Design review of the part built by this model. Coordinates are the model's own, in mm. A direction names the side the tool comes from. Coordinates: 2 decimals unless noted, no trailing zeros. Write each loop counter-clockwise with the first axis right and the second up, starting at its lowest first coordinate (ties: lowest second). Pieces come first, ordered by that corner, then holes. Notation, with made-up numbers: (-18, 43) -> (-10, 43) arc R20 ccw to (-10, 49) -> close; hole circle Ø1 at (7, -6.5). An arc over 180 degrees is marked (long way). Answer in a Markdown table with one row per item. Add a question column.
Item 1: Take a section at A-A, the plane z = -6.5. Write out the cut boundary in (x, y), and give its area (3 significant figures).
Item 2: Draft analysis for pull direction X (two halves, no side actions). For faces 4 (the face through (18.374, 39, 14)), 5 (the face through (20.374, 21, 16)), 6 (the face through (0.4, 80, -8.3)), 7 (the face through (1, 39, -7.879)), state which applies: released by +X, released by -X, zero draft, split by the parting line, or undercut.
Item 3: For faces 1 (the face through (19.39, 24.35, 11.92)), 2 (the face through (-17.283, 39, 13)), 3 (the face through (-24.283, 39, 10)), list the 3-axis set-ups (+Z, -Z, +X, -X, +Y, -Y) from which the entire face can be reached by the end or side of a thin tool; tool diameter is ignored.
Item 4: Clearance check with flat-ended pins moving along their axes: P1, Ø10.5, axis at x = -4, y = 24.5, coming from the +Z side; P2, Ø7.5, axis at y = 18, z = 13.5, coming from the +X side; P3, Ø9, axis at y = 18.63, z = 10.12, coming from the +X side. State where each tip first meets the part, or that it passes through.
Item 5: Take a section at C-C, the plane x = -7. Write out the cut boundary in (y, z), and give its area (3 significant figures).
Item 6: To check wall thickness, follow line 1 (X direction, y = 51, z = 9); line 2 (Z direction, x = -2.5, y = 8). State the ranges of each line that lie inside material, in increasing order.
Item 7: Take a section at B-B, the plane y = 32.5. Write out the cut boundary in (x, z), and give its area (3 significant figures).
from build123d import *

# Parameters (mm, degrees)
F1_DEPTH = 80
F2_R     = 6
F3_DEPTH = 25
F2_R_2   = 7.5
F4_DEPTH = 5


with BuildPart() as f1:
    # F0 (on Front) → F1 (new body)
    with BuildSketch(Plane.XZ):
        Polygon((-17.282601, 35.120948), (-24.282601, 35.120948), (-24.282601, -14.879052), (25.373651, -14.879052), (25.373651, 35.120948), (18.373651, 35.120948), (18.373651, -7.879052), (-17.282601, -7.879052), align=None)
    extrude(amount=-F1_DEPTH)

    # F2 (on face) → F3 (cut)
    with BuildSketch(Plane.YZ.offset(25.373651)):
        with Locations((18.626541, 10.120948)):
            Circle(F2_R)
    extrude(amount=-F3_DEPTH, mode=Mode.SUBTRACT)

    # F2 (on face) → F4 (cut)
    with BuildSketch(Plane.YZ.offset(25.373651)):
        with Locations((18.626541, 10.120948)):
            Circle(F2_R_2)
        with Locations((18.626541, 10.120948)):
            Circle(F2_R, mode=Mode.SUBTRACT)
    extrude(amount=-F4_DEPTH, mode=Mode.SUBTRACT)


solid = f1.part
Answers:
| question | item | result |
|---|---|---|
| 1 | outline | (-24.28, 0) -> (-17.28, 0) -> (-17.28, 80) -> (-24.28, 80) -> close; (18.37, 0) -> (25.37, 0) -> (25.37, 80) -> (18.37, 80) -> close |
| 1 | area | 1,120 mm^2 |
| 2 | face 4 | undercut |
| 2 | face 5 | released by +X |
| 2 | face 6 | zero draft |
| 2 | face 7 | undercut |
| 3 | face 1 | +X |
| 3 | face 2 | +Z, +Y, -Y |
| 3 | face 3 | +Z, -Z, -X, +Y, -Y |
| 4 | P1 | stops at z = -7.88 |
| 4 | P2 | stops at x = 20.37 |
| 4 | P3 | stops at x = -17.28 |
| 5 | outline | (0, -14.88) -> (80, -14.88) -> (80, -7.88) -> (0, -7.88) -> close |
| 5 | area | 560 mm^2 |
| 6 | line 1 | x = -24.28 to -17.28, 18.37 to 25.37 |
| 6 | line 2 | z = -14.88 to -7.88 |
| 7 | outline | (-24.28, -14.88) -> (25.37, -14.88) -> (25.37, 35.12) -> (18.37, 35.12) -> (18.37, -7.88) -> (-17.28, -7.88) -> (-17.28, 35.12) -> (-24.28, 35.12) -> close |
| 7 | area | 950 mm^2 |
